Work out the finished part from the listing and answer in its coordinate system (mm). A direction names the side the tool comes from. Give positions to 0.01 mm unless a question says otherwise; leave off trailing zeros. Loops run counter-clockwise (first coordinate to the right, second up) from the corner with the lowest first, then second, coordinate; pieces in that order, holes last. Notation, with made-up numbers: M -32,70 L 11,70 A21 cw 11,78 Z; hole C 73.25,71.5 d9. An arc over 180 degrees is marked long. Write item = value, one per line. Start each with the question number.
1. For faces 4 (the face through (-3.175, 48, 0)), 5 (the face through (13, 55, 1.27)), 6 (the face through (16, -14, -7.821)), determine the directions among +Z, -Z, +X, -X, +Y, -Y from which every point of the face is accessible in a straight line to the end or side of a thin tool.
2. The mould has two halves that part along Y. Classify faces 1 (the face through (6.883, 3.131, 30.995)), 2 (the face through (13.02, 63.82, 0.02)), 3 (the face through (-5.94, 50.05, 0.02)): released by +Y, released by -Y, zero draft, split by the parting line, or undercut.
3. Section A-A on x = -6 is taken. Determine the outline of the cut face in (y, z), plus the area to 3 significant figures.
4. Consider L1, parallel to Z at x = 0, y = 4; L2, parallel to Y at x = -7.5, z = -11; L3, parallel to Y at x = 11.5, z = 23.5. Determine where each line is inside the solid, lowest interval first. Write a range as [from, to].
5. Section B-B on z = -19 is taken. Determine the outline of the cut face in (x, y).
6. Flat-ended cylindrical pins translate along their axes: pin 1 Ø2 at (y, z) = (46.5, 0.5) entering from +X; pin 2 Ø5 at (y, z) = (-1, -17.5) entering from -X; pin 3 Ø2 at (y, z) = (47, 0.5) entering from -X (3 decimals). Find the tip coordinate at first contact, or state that the pin passes through.
7. Section C-C on y = -11.5 is taken. Determine the outline of the cut face in (x, z).
8. Section D-D on x = -24.5 is taken. Determine the outline of the cut face in (y, z), plus the area to 3 significant figures.
Autodesk Inventor part; units mm, degrees
ref_plane "YZ Plane" through (0, 0, 0) normal (1, 0, 0) x (0, 1, 0)
ref_plane "XZ Plane" through (0, 0, 0) normal (0, 1, 0) x (-1, 0, 0)
ref_plane "XY Plane" through (0, 0, 0) normal (0, 0, 1) x (1, 0, 0)
sketch "Sketch1" plane through (0, 0, 0) normal (0, 1, 0) x (-1, 0, 0)
  circle A0 centre (0, 0) radius 31.75
  dimension "d0" = 63.5
extrude "Extrusion1" add sketch "Sketch1" along normal blind 6.35
sketch "Sketch3" plane through (0, 6.35, 0) normal (0, 1, 0) x (1, 0, 0)
  circle A0 centre (0, 0) radius 12.7
  dimension "d9" = 25.4
extrude "Extrusion3" add sketch "Sketch3" along normal blind 31.75
sketch "Sketch4" plane through (0, 38.1, 0) normal (0, 1, 0) x (1, 0, 0)
  circle A0 centre (0, 0) radius 14.9177
extrude "Extrusion4" add sketch "Sketch4" along normal blind 7.62
sketch "Sketch5" plane through (0, 45.72, 0) normal (0, 1, 0) x (1, 0, 0)
  line L0 (-3.175, 1.27) -> (3.175, 1.27)
  line L1 (3.175, 1.27) -> (3.175, -1.27)
  line L2 (3.175, -1.27) -> (-3.175, -1.27)
  line L3 (-3.175, -1.27) -> (-3.175, 1.27)
  line L4 (-3.175, 1.27) -> (3.175, -1.27) construction
  line L5 (3.175, 1.27) -> (-3.175, -1.27) construction
  point P0 (0, 0)
  dimension "d14" = 6.35
  dimension "d15" = 2.54
extrude "Extrusion5" add sketch "Sketch5" along normal blind 2.54
sketch "Sketch6" plane through (-3.175, 45.72, 1.27) normal (0, 0, 1) x (1, 0, 0)
  line L0 (-8.0078, 1.2174) -> (37.195, 1.2174)
  line L1 (40.37, 4.3924) -> (40.37, 15.4306)
  line L2 (37.195, 18.6056) -> (-8.0078, 18.6056)
  line L3 (-8.0078, 12.7012) -> (-8.0078, 7.9542)
  arc A0 (37.195, 1.2174) -> (40.37, 4.3924) centre (37.195, 4.3924) ccw
  arc A1 (40.37, 15.4306) -> (37.195, 18.6056) centre (37.195, 15.4306) ccw
  arc A2 (-5.4455, 4.8388) -> (37.195, 1.2174) centre (32.3527, 197.046) ccw
  arc A3 (37.195, 18.6056) -> (-5.2937, 15.8426) centre (33.0266, -245.3603) ccw
  arc A4 (-8.0078, 7.9542) -> (-5.4455, 4.8388) centre (-4.8328, 7.9542) ccw
  arc A5 (-5.2937, 15.8426) -> (-8.0078, 12.7012) centre (-4.8328, 12.7012) ccw
  line L4 (0, 2.54) -> (0, 3.8476)
  line L5 (6.35, 2.54) -> (0, 2.54)
  line L6 (6.35, 2.54) -> (6.35, 2.891)
  arc A6 (0, 3.8476) -> (6.35, 2.891) centre (32.3527, 197.046) ccw
  point P0 (3.175, -45.72)
  point P1 (-8.0078, 5.3605)
  point P2 (-8.0078, 15.43)
  dimension "d18" = 3.175
  dimension "d19" = 3.175
extrude "Extrusion6" add sketch "Sketch6" against normal blind 2.54
sketch "Sketch7" plane through (0, 45.72, 0) normal (0, 1, 0) x (1, 0, 0)
  circle A0 centre (0, 0) radius 13.5422
  circle A1 centre (0, 0) radius 14.9177
extrude "Extrusion7" cut sketch "Sketch7" against normal blind 25.4
sketch "Sketch8" plane through (0, 0, 0) normal (0, -1, 0) x (1, 0, 0)
  circle A0 centre (0, 0) radius 29.6911
  circle A1 centre (0, 0) radius 8.89
  line L0 (-4.226, 7.8213) -> (-28.6424, 7.8213)
  line L1 (4.226, 7.8213) -> (28.6424, 7.8213)
  line L2 (4.226, -7.8213) -> (28.6424, -7.8213)
  line L3 (-4.226, -7.8213) -> (-28.6424, -7.8213)
  arc A2 (-28.6424, 7.8213) -> (-28.6424, -7.8213) centre (0, 0) ccw
  arc A3 (28.6424, -7.8213) -> (28.6424, 7.8213) centre (0, 0) ccw
  dimension "d24" = 17.78
extrude "Extrusion8" add sketch "Sketch8" along normal blind 29.3624 contours A0 L2 A1 L1 | L0 A1 L3 A0 | A1
sketch "Sketch10" plane through (0, 0, 0) normal (0, -1, 0) x (1, 0, 0)
  circle A0 centre (0, 0) radius 31.75
  line L0 (0, -31.75) -> (0, -19)
  line L1 (0, -19) -> (0, 31.75)
  line L2 (0, 31.75) -> (0, 19)
  circle A1 centre (0, 19) radius 2.921
  circle A2 centre (0, -19) radius 2.921
  dimension "d31" = 12.75
  dimension "d32" = 12.75
  dimension "d33" = 5.842
extrude "Extrusion9" cut sketch "Sketch10" against normal blind 25.4 contours A1 L1 | L1 A1 | A2 L1 L0 | L0 L1 A2
properties part number "masterswitch"
Verdict:
q1.face_4 = +Z, -Z, -X
q1.face_5 = +Z, +X, -X, +Y
q1.face_6 = -Z, +X, -Y
q2.face_1 = zero draft
q2.face_2 = released by +Y
q2.face_3 = undercut
q3.outline = M -29.36,-7.82 L 0,-7.82 L 0,-31.18 L 6.35,-31.18 L 6.35,-11.19 L 38.1,-11.19 L 38.1,-12.14 L 45.72,-12.14 L 45.72,12.14 L 38.1,12.14 L 38.1,11.19 L 6.35,11.19 L 6.35,31.18 L 0,31.18 L 0,7.82 L -29.36,7.82 Z; M 50.06,-1.27 L 61.91,-1.27 L 61.91,1.27 L 50.06,1.27 Z
q3.area = 1,780 mm2
q4.L1 = [-31.75, -21.92], [-16.08, 16.08], [21.92, 31.75]
q4.L2 = [0, 6.35], [38.1, 45.72]
q4.L3 = [0, 6.35]
q5.outline = M -25.44,0 L -2.92,0 L -2.92,6.35 L -25.44,6.35 Z; M 2.92,0 L 25.44,0 L 25.44,6.35 L 2.92,6.35 Z
q6.pin_1 = 35.82
q6.pin_2 = -27.87
q6.pin_3 = -3.175
q7.outline = M -28.64,-7.82 L -4.23,-7.82 A8.89 ccw 4.23,-7.82 L 28.64,-7.82 A29.69 ccw 28.64,7.82 L 4.23,7.82 A8.89 ccw -4.23,7.82 L -28.64,7.82 A29.69 ccw Z
q8.outline = M -29.36,-7.82 L 0,-7.82 L 0,-20.19 L 6.35,-20.19 L 6.35,20.19 L 0,20.19 L 0,7.82 L -29.36,7.82 Z
q8.area = 716 mm2
